```python
from build123d import *

# Parameters (mm, degrees)
SKETCH_1_W          = 95
SKETCH_1_H          = 45.5
EXTRUDE_1_DEPTH     = 2
SKETCH_2_W          = 7
SKETCH_2_H          = 2
CUT_EXTRUDE_1_DEPTH = 106.352978126
SKETCH_3_R          = 0.5
CUT_EXTRUDE_2_DEPTH = 106.352978126
SKETCH_5_W          = 13.5
SKETCH_5_H          = 24.5
CUT_EXTRUDE_3_DEPTH = 106.352978126
SKETCH_6_W          = 2
SKETCH_6_H          = 7
EXTRUDE_2_DEPTH     = 2
SKETCH_7_W          = 20
SKETCH_7_H          = 12
CUT_EXTRUDE_4_DEPTH = 108.159927212
CUT_EXTRUDE_5_DEPTH = 108.159927212
FILLET_1_R          = 1
SKETCH_9_R          = 1.6
CUT_EXTRUDE_6_DEPTH = 2


with BuildPart() as part:
    # 草图1 → 凸台-拉伸1 (new body)
    with BuildSketch(Plane.XY):
        with Locations((47.5, 22.75)):
            Rectangle(SKETCH_1_W, SKETCH_1_H)
    extrude(amount=EXTRUDE_1_DEPTH)

    # 草图2 → 切除-拉伸1 (cut, through all)
    with BuildSketch(Plane.XY.offset(2)):
        with Locations((58.5, 44.5)):
            Rectangle(SKETCH_2_W, SKETCH_2_H)
        with Locations((36.5, 44.5)):
            Rectangle(SKETCH_2_W, SKETCH_2_H)
        with Locations((14.5, 44.5)):
            Rectangle(SKETCH_2_W, SKETCH_2_H)
        with Locations((36.5, 1)):
            Rectangle(SKETCH_2_W, SKETCH_2_H)
        with Locations((58.5, 1)):
            Rectangle(SKETCH_2_W, SKETCH_2_H)
        with Locations((80.5, 1)):
            Rectangle(SKETCH_2_W, SKETCH_2_H)
    extrude(amount=-CUT_EXTRUDE_1_DEPTH, mode=Mode.SUBTRACT)

    # 草图3 → 切除-拉伸2 (cut, through all)
    with BuildSketch(Plane.XY.offset(2)):
        with Locations((11, 43.5)):
            Circle(SKETCH_3_R)
    cut_extrude_2 = extrude(amount=-CUT_EXTRUDE_2_DEPTH, mode=Mode.SUBTRACT)

    # 草图5 → 切除-拉伸3 (cut, through all)
    with BuildSketch(Plane.XY.offset(2)):
        with Locations((6.75, 12.25)):
            Rectangle(SKETCH_5_W, SKETCH_5_H)
    extrude(amount=-CUT_EXTRUDE_3_DEPTH, mode=Mode.SUBTRACT)

    # 草图6 → 凸台-拉伸2 (add)
    with BuildSketch(Plane.XY.offset(2)):
        with Locations((-1, 35)):
            Rectangle(SKETCH_6_W, SKETCH_6_H)
        with Locations((96, 32)):
            Rectangle(SKETCH_6_W, SKETCH_6_H)
        with Locations((96, 13.5)):
            Rectangle(SKETCH_6_W, SKETCH_6_H)
    extrude(amount=-EXTRUDE_2_DEPTH)

    # 草图阵列1: 切除-拉伸2 at 17 more places
    with Locations((7, 0, 0), (22, 0, 0), (29, 0, 0), (44, 0, 0), (51, 0, 0), (73, -41.5, 0), (66, -41.5, 0), (51, -41.5, 0), (44, -41.5, 0), (29, -41.5, 0), (22, -41.5, 0), (-11, -12, 0), (84, -8, 0), (-11, -5, 0), (84, -15, 0), (84, -26.5, 0), (84, -33.5, 0)):
        add(cut_extrude_2, mode=Mode.SUBTRACT)

    # 草图7 → 切除-拉伸4 (cut, through all)
    with BuildSketch(Plane(origin=(0, 0, 0), x_dir=(-1, 0, 0), z_dir=(0, 0, -1))):
        with Locations((-81, 12)):
            Rectangle(SKETCH_7_W, SKETCH_7_H)
    extrude(amount=-CUT_EXTRUDE_4_DEPTH, mode=Mode.SUBTRACT)

    # 草图8 → 切除-拉伸5 (cut, through all)
    with BuildSketch(Plane(origin=(0, 0, 0), x_dir=(-1, 0, 0), z_dir=(0, 0, -1))):
        Polygon((-91, 7.5), (-95, 1.5), (-95, 0), (-93.5, 0), (-89.5, 6), (-91, 6), align=None)
    extrude(amount=-CUT_EXTRUDE_5_DEPTH, mode=Mode.SUBTRACT)

    # 圆角1
    fillet_1_edges = [part.edges().sort_by_distance(p)[0] for p in [
        (91, 7.5, 1),
        (89.5, 6, 1),
        (93.5, 0, 1),
        (95, 1.5, 1),
    ]]
    fillet(fillet_1_edges, radius=FILLET_1_R)

    # 草图9 → 切除-拉伸6 (cut)
    with BuildSketch(Plane(origin=(0, 0, 0), x_dir=(-1, 0, 0), z_dir=(0, 0, -1))):
        with Locations((-6.75, 40.5)):
            Circle(SKETCH_9_R)
        with Locations((-22.75, 13)):
            Circle(SKETCH_9_R)
    extrude(amount=-CUT_EXTRUDE_6_DEPTH, mode=Mode.SUBTRACT)


solid = part.part
```
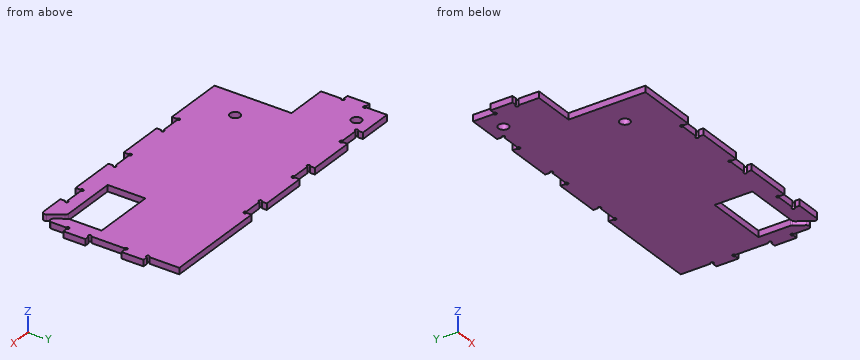
Geometry check sheet. Reference: the model listing, model coordinates, mm. Give positions to 0.01 mm unless a question says otherwise; leave off trailing zeros. Order: outer loops, then holes, each group sorted by start corner. A loop starts at its lowest first (then second) coordinate and runs counter-clockwise, first axis right, second up. Notation, with made-up numbers: (9.25, 21.5) - (25.25, 21.5) arc R24 cw to (25.25, 49.5) - close; hole circle Ø8 at (86.5, 49). An arc over 180 degrees is marked (long way). Answer in a Markdown table with one row per item. Add a question column.
Q1. Cross-section at A-A, the plane x = 22.75. Enter the section's corners in (y, z), then the cut area to 3 significant figures.
Q2. Cross-section at B-B, the plane z = 0.3. Count the separate pieces of the cut face and the enclosed holes in it, then the cut area to 3 significant figures.
Q3. Cross-section at C-C, the plane x = 35. Enter the section's corners in (y, z).
Q4. Cross-section at D-D, the plane y = 22.5. Enter the section's corners in (x, z), then the cut area to 3 significant figures.
Q5. Material ranges on probe 1 along Y at (x, z) = (87.5, 1.6); probe 2 along X at (y, z) = (14, 1.2); probe 3 along Y at (x, z) = (22.75, 1.3), recorded low to high. Write a range as from..to.
Q6. Gauge pin test, flat ends, axial feed: pin 1 (0.6 mm diameter, centred on x = 37.5, z = 1.5, fed in from -Y); pin 2 (0.8 mm diameter, centred on y = 0.5, z = 1, fed in from -X); pin 3 (1.2 mm diameter, centred on y = 44.5, z = 1, fed in from -X). Record the tip position at first contact, or that the pin passes through.
Check values:
| question | item | result |
|---|---|---|
| 1 | outline | (0, 0) - (11.4, 0) - (11.4, 2) - (0, 2) - close; (14.6, 0) - (45.5, 0) - (45.5, 2) - (14.6, 2) - close |
| 1 | area | 84.6 mm^2 |
| 2 | separate pieces | 1 |
| 2 | enclosed holes | 2 |
| 2 | area | 3,670 mm^2 |
| 3 | outline | (2, 0) - (43.5, 0) - (43.5, 2) - (2, 2) - close |
| 4 | outline | (13.5, 0) - (95, 0) - (95, 2) - (13.5, 2) - close |
| 4 | area | 163 mm^2 |
| 5 | probe 1 | y = 0..6, 18..45.5 |
| 5 | probe 2 | x = 13.5..21.5, 24..71, 91..97 |
| 5 | probe 3 | y = 0..11.4, 14.6..45.5 |
| 6 | pin 1 | stops at y = 2 |
| 6 | pin 2 | stops at x = 13.5 |
| 6 | pin 3 | stops at x = 0 |
